```python
from build123d import *

# Parameters (mm, degrees)
SKETCH3_W           = 80
SKETCH3_H           = 80
BOSS_EXTRUDE1_DEPTH = 3
FILLET3_R           = 20
FILLET4_R           = 20
FILLET5_R           = 20
FILLET6_R           = 20
SKETCH6_R           = 1.5
CUT_EXTRUDE2_DEPTH  = 3
SKETCH9_R           = 1.5
CUT_EXTRUDE3_DEPTH  = 3
SKETCH12_R          = 1.5
CUT_EXTRUDE6_DEPTH  = 3
SKETCH13_R          = 1.5
CUT_EXTRUDE7_DEPTH  = 3
SKETCH14_W          = 20
SKETCH14_H          = 5
CUT_EXTRUDE8_DEPTH  = 10


with BuildPart() as part:
    # Sketch3 → Boss-Extrude1 (new body)
    with BuildSketch(Plane(origin=(0, 0, 0), x_dir=(1, 0, 0), z_dir=(0, 1, 0))):
        with Locations((40, 40)):
            Rectangle(SKETCH3_W, SKETCH3_H)
    extrude(amount=BOSS_EXTRUDE1_DEPTH)

    # Fillet3
    fillet3_edges = [part.edges().sort_by_distance(p)[0] for p in [
        (0, 1.5, -80),
    ]]
    fillet(fillet3_edges, radius=FILLET3_R)

    # Fillet4
    fillet4_edges = [part.edges().sort_by_distance(p)[0] for p in [
        (80, 1.5, -80),
    ]]
    fillet(fillet4_edges, radius=FILLET4_R)

    # Fillet5
    fillet5_edges = [part.edges().sort_by_distance(p)[0] for p in [
        (80, 1.5, 0),
    ]]
    fillet(fillet5_edges, radius=FILLET5_R)

    # Fillet6
    fillet6_edges = [part.edges().sort_by_distance(p)[0] for p in [
        (0, 1.5, 0),
    ]]
    fillet(fillet6_edges, radius=FILLET6_R)

    # Sketch6 → Cut-Extrude2 (cut)
    with BuildSketch(Plane(origin=(0, 3, 0), x_dir=(1, 0, 0), z_dir=(0, 1, 0))):
        with Locations((17, 58.5)):
            Circle(SKETCH6_R)
        with Locations((62, 58.5)):
            Circle(SKETCH6_R)
    extrude(amount=-CUT_EXTRUDE2_DEPTH, mode=Mode.SUBTRACT)

    # Sketch9 → Cut-Extrude3 (cut)
    with BuildSketch(Plane(origin=(0, 3, 0), x_dir=(1, 0, 0), z_dir=(0, 1, 0))):
        with Locations((70, 10)):
            Circle(SKETCH9_R)
        with Locations((10, 10)):
            Circle(SKETCH9_R)
    extrude(amount=-CUT_EXTRUDE3_DEPTH, mode=Mode.SUBTRACT)

    # Sketch12 → Cut-Extrude6 (cut)
    with BuildSketch(Plane(origin=(0, 3, 0), x_dir=(1, 0, 0), z_dir=(0, 1, 0))):
        with Locations((30, 5)):
            Circle(SKETCH12_R)
        with Locations((50, 5)):
            Circle(SKETCH12_R)
    extrude(amount=-CUT_EXTRUDE6_DEPTH, mode=Mode.SUBTRACT)

    # Sketch13 → Cut-Extrude7 (cut)
    with BuildSketch(Plane(origin=(0, 3, 0), x_dir=(1, 0, 0), z_dir=(0, 1, 0))):
        with Locations((20, 70)):
            Circle(SKETCH13_R)
        with Locations((60, 70)):
            Circle(SKETCH13_R)
    extrude(amount=-CUT_EXTRUDE7_DEPTH, mode=Mode.SUBTRACT)

    # Sketch14 → Cut-Extrude8 (cut)
    with BuildSketch(Plane(origin=(0, 3, 0), x_dir=(1, 0, 0), z_dir=(0, 1, 0))):
        with Locations((40, 57.5)):
            Rectangle(SKETCH14_W, SKETCH14_H)
        with Locations((40, 20.5)):
            Rectangle(SKETCH14_W, SKETCH14_H)
    extrude(amount=-CUT_EXTRUDE8_DEPTH, mode=Mode.SUBTRACT)


solid = part.part
```
Geometry check sheet. Reference: the model listing, model coordinates, mm. A direction names the side the tool comes from. Give positions to 0.01 mm unless a question says otherwise; leave off trailing zeros. Write each loop counter-clockwise with the first axis right and the second up, starting at its lowest first coordinate (ties: lowest second). Pieces come first, ordered by that corner, then holes.
1) Material ranges on L1, parallel to Z at x = 45.5, y = 0.15; L2, parallel to X at y = 2, z = -70; L3, parallel to X at y = 1.7, z = -55.5, recorded low to high.
2) Section check C-C, the plane x = 36. Record the boundary of the cut face in (y, z), and give its area (3 significant figures).
3) Section check B-B, the plane x = 17. Record the boundary of the cut face in (y, z), and give its area (3 significant figures).
4) Access from +Z, -Z, +X, -X, +Y, -Y to the whole of each face (thin tool, end or side, straight path). Record for faces 4 (the flat face through (39, 0, -41)), 5 (the flat face through (30, 2, -57)).
5) Gauge pin test, flat ends, axial feed: pin 1 (3.5 mm diameter, centred on x = 60, z = -70, fed in from +Y); pin 2 (1.8 mm diameter, centred on x = 70, z = -10, fed in from +Y). Record the tip position at first contact, or that the pin passes through.
6) Section check A-A, the plane y = 1.05. State how many separate pieces and enclosed holes the cut face has, and give its area (3 significant figures).
7) Release check for a two-part mould opening along Z. For faces 1 (the flat face through (39, 3, -41)), 2 (the flat face through (40, 2, -55)), 3 (the cylindrical face through (74.297, 1.521, -6.014)) record: pulls with the +Z half, pulls with the -Z half, needs draft (parallel to the pull), parting line crosses it, or undercut.
Computed:
1. L1: z = -80 to -60, -55 to -23, -18 to 0
1. L2: x = 2.68 to 18.5, 21.5 to 58.5, 61.5 to 77.32
1. L3: x = 0 to 30, 50 to 80
2. outline: (0, -80) - (3, -80) - (3, -60) - (0, -60) - close; (0, -55) - (3, -55) - (3, -23) - (0, -23) - close; (0, -18) - (3, -18) - (3, 0) - (0, 0) - close
2. area: 210 mm2
3. outline: (0, -79.77) - (3, -79.77) - (3, -60) - (0, -60) - close; (0, -57) - (3, -57) - (3, -0.23) - (0, -0.23) - close
3. area: 230 mm2
4. face 4: +Z, -Z, +X, -X, -Y
4. face 5: +Y, -Y
5. pin 1: stops at y = 3
5. pin 2: passes through
6. separate pieces: 1
6. enclosed holes: 10
6. area: 5,800 mm2
7. face 1: needs draft
7. face 2: undercut
7. face 3: pulls with the +Z half
